For this review, take the finished solid that the model builds, in its own axes (mm). Give positions to 0.01 mm unless a question says otherwise; leave off trailing zeros. Order: outer loops, then holes, each group sorted by start corner. A loop starts at its lowest first (then second) coordinate and runs counter-clockwise, first axis right, second up. Notation, with made-up numbers: (0.25, -8.75) -> (31.25, -8.75) arc R23 cw to (31.25, 9.25) -> close; hole circle Ø8 at (-3, -30). An arc over 180 degrees is marked (long way). One line per item, written item: value. Start each with the question number.
from build123d import *

# Parameters (mm, degrees)
F0_W           = 100
F0_H           = 80
F1_DEPTH       = 50
F3_D           = 5.11
F3_CBORE_D     = 11.11
F3_CBORE_DEPTH = 6.35


with BuildPart() as f1:
    # F0 (on Top) → F1 (new body)
    with BuildSketch(Plane.XY):
        with Locations((0.469463, 24.830001)):
            Rectangle(F0_W, F0_H)
    extrude(amount=F1_DEPTH)

    # F3 (through all)
    with Locations(Plane.XY.offset(50)):
        with Locations((-31.00967, 37.677433), (18.126821, 23.215853)):
            CounterBoreHole(F3_D / 2, F3_CBORE_D / 2, F3_CBORE_DEPTH)


solid = f1.part
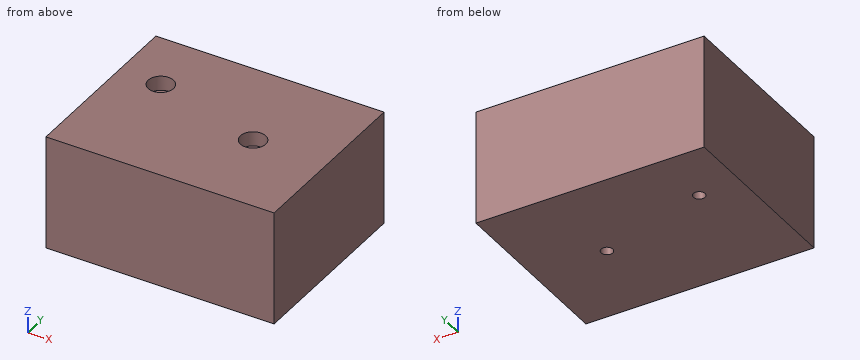
Q1. For line 1 along X through (y, z) = (21, 44.5); line 2 along Y through (x, z) = (-30.5, 30); line 3 along Y through (x, z) = (19.5, 46.5), list the stretches that pass through material, from the lowest coordinate up.
Q2. For pin 1 Ø10 at (x, y) = (-31.01, 37.68) entering from +Z, flat-tipped, find the tip position at first contact; note if it passes through.
Q3. Take a section at A-A (z = 46.5). State the section outline as (x, y) points (3 decimals).
Answers below:
1. line 1: x = -49.53 to 13.03, 23.22 to 50.47
1. line 2: y = -15.17 to 35.17, 40.18 to 64.83
1. line 3: y = -15.17 to 17.83, 28.6 to 64.83
2. pin 1: stops at z = 43.65
3. outline: (-49.531, -15.17) -> (50.469, -15.17) -> (50.469, 64.83) -> (-49.531, 64.83) -> close; hole circle Ø11.11 at (-31.01, 37.677); hole circle Ø11.11 at (18.127, 23.216)
